Model file for the job. Use its own axes, mm. Round coordinates to 2 decimals unless told otherwise and drop trailing zeros. Loops run counter-clockwise (first coordinate to the right, second up) from the corner with the lowest first, then second, coordinate; pieces in that order, holes last. Notation, with made-up numbers: M -40,59.5 L -23,59.5 A24 cw -23,80.5 Z; hole C -4,83 d5. An arc over 180 degrees is marked long. Use a Markdown table: item, result. Add a question column.
Q1. Mould opens along Y. For faces 1 (the face through (14.27, 3.71, 1.98)), 2 (the face through (11, 8, 2)), 3 (the face through (21, 3.9, 0.5)) say: +Y half, -Y half, draft (parallel to the pull), parting line (faces both ways), or undercut.
Q2. Probe line 1 (X direction, y = 3, z = 1.2); line 2 (X direction, y = 2.5, z = 2); line 3 (Y direction, x = 16.5, z = 2.3). List the from-to ranges inside material, lowest first. Write a range as from..to.
Q3. Cut at D-D (x = 6.25). Give the cut face in (y, z).
Q4. Pin check, flat tips, straight feed: pin 1 (1.2 mm diameter, centred on x = 7.5, y = 6.5, fed in from +Z); pin 2 (3 mm diameter, centred on x = 17, y = 1, fed in from +Z); pin 3 (3 mm diameter, centred on y = 1, z = 4, fed in from +X). Stop position of each tip, or through.
Q5. Cut at C-C (z = 2.8). Give the cut face in (x, y), plus the area to 3 significant figures.
Q6. Cut at A-A (y = 4). Give the cut face in (x, z).
Q7. Cut at B-B (x = 16.5). Give the cut face in (y, z).
Autodesk Inventor part; units mm, degrees
ref_plane "Work Plane2" through (10.5, 0, 0) normal (-1, 0, 0) x (0, 0, 1)
ref_plane "YZ Plane" through (0, 0, 0) normal (1, 0, 0) x (0, 1, 0)
ref_plane "XZ Plane" through (0, 0, 0) normal (0, 1, 0) x (-1, 0, 0)
sketch "Sketch1" plane through (0, 0, 0) normal (0, 0, 1) x (1, 0, 0)
  line L0 (0, 0) -> (21, 0)
  line L1 (21, 0) -> (21, 8)
  line L2 (21, 8) -> (0, 8)
  line L3 (0, 8) -> (0, 0)
  dimension "d0" = 21
  dimension "d1" = 8
extrude "Extrusion1" add sketch "Sketch1" along normal blind 4
sketch "Sketch2" plane through (0, 8, 0) normal (0, 1, 0) x (1, 0, 0)
  line L0 (0, 0) -> (0, -4)
  line L1 (0, -4) -> (21, -4)
  arc A0 (3, -4) -> (0, -1) centre (-0.8979, -4.8979) ccw
  line L2 (21, 0) -> (21, -4)
  arc A1 (21, -1) -> (18, -4) centre (21.8979, -4.8979) ccw
  dimension "d4" = 4
  dimension "d5" = 1
  dimension "d6" = 3
  dimension "d7" = 3
extrude "Extrusion2" cut sketch "Sketch2" against normal up to next
ref_plane "Work Plane2" through (10.5, 0, 0) normal (-1, 0, 0) x (0, 0, 1)
sketch "Sketch5" plane through (10.5, 0, 0) normal (-1, 0, 0) x (0, 0, 1)
  line L0 (4, 8) -> (4, 0)
  line L1 (4, 0) -> (4, 8)
  arc A0 (4, 2) -> (4, 6) centre (2.5, 4) ccw
  point P0 (0, 0)
  dimension "d25" = 2.5
  dimension "d26" = 1.5
  dimension "d27" = 4
extrude "Extrusion4" add sketch "Sketch5" along normal mid plane 12
sketch "Sketch3" plane through (0, 0, 0) normal (0, 0, -1) x (-1, 0, 0)
  line L0 (-21, 8) -> (0, 8)
  line L1 (-21, 0) -> (-21, 8)
  point P0 (-4.5, 4)
  point P1 (-16.5, 4)
  dimension "d10" = 12
  dimension "d11" = 4.5
  dimension "d12" = 4
hole "Hole1" at (4.5, 4, 0) at (16.5, 4, 0) direction (0, 0, 1) diameter 4.5 end through all
properties part number "Infill3DLever"
Checked values:
| question | item | result |
|---|---|---|
| 1 | face 1 | undercut |
| 1 | face 2 | +Y half |
| 1 | face 3 | draft |
| 2 | line 1 | x = 0.63..2.48, 6.52..14.48, 18.52..20.37 |
| 2 | line 2 | x = 1.86..2.82, 6.18..14.82, 18.18..19.14 |
| 2 | line 3 | y = 0..1.75, 6.25..8 |
| 3 | outline | M 0,0 L 2.59,0 L 2.59,4.56 A2.5 ccw 2,4 L 0,4 Z; M 5.41,0 L 8,0 L 8,4 L 6,4 A2.5 ccw 5.41,4.56 Z |
| 4 | pin 1 | stops at z = 4.12 |
| 4 | pin 2 | stops at z = 4 |
| 4 | pin 3 | stops at x = 18.7 |
| 5 | outline | M 2.51,0 L 18.49,0 L 18.49,2.95 A2.25 cw long 18.49,5.05 L 18.49,8 L 2.51,8 L 2.51,5.05 A2.25 cw long 2.51,2.95 Z |
| 5 | area | 96.8 mm^2 |
| 6 | outline | M 0,0 L 2.25,0 L 2.25,2.43 A4 cw 0,1 Z; M 6.75,0 L 14.25,0 L 14.25,5 L 6.75,5 Z; M 18.75,0 L 21,0 L 21,1 A4 cw 18.75,2.43 Z |
| 7 | outline | M 0,0 L 1.75,0 L 1.75,4 L 0,4 Z; M 6.25,0 L 8,0 L 8,4 L 6.25,4 Z |
